Geometry: see drawing. Coordinates: mm, zero at the bounding-box minimum. Coordinates: 2 decimals unless noted, no trailing zeros. Order: outer loops, then holes, each group sorted by start corner. A loop starts at its lowest first (then second) coordinate and runs counter-clockwise, first axis right, second up.
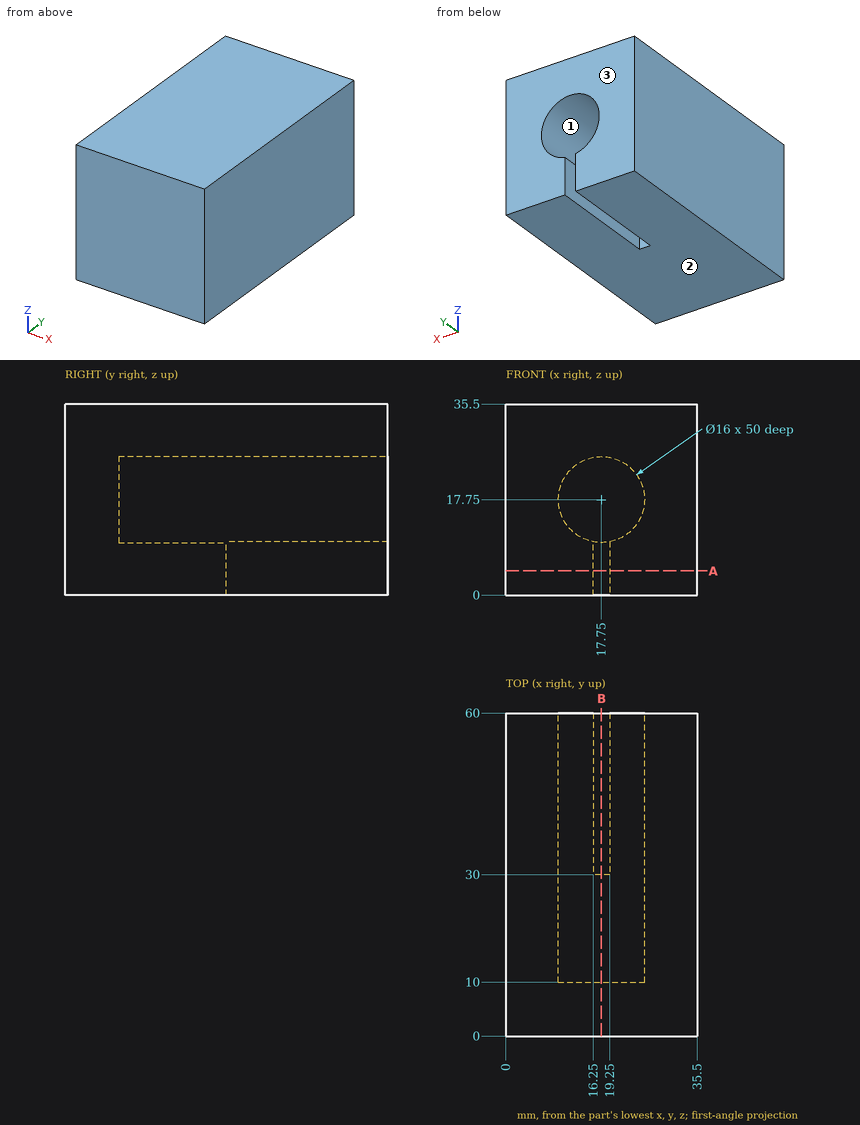
Q1. Section query B-B on x = 17.75. Output: boundary loops of the cut face in (y, z).
Solutions:
outline: (0, 0) - (30, 0) - (30, 9.75) - (10, 9.75) - (10, 25.75) - (60, 25.75) - (60, 35.5) - (0, 35.5) - close
Q2. Pull-direction query (Z, two-part tool) for the marked faces 1, 2 and 3; classes: pulls with the +Z half, pulls with the -Z half, needs draft (parallel to the pull), parting line crosses it, or undercut.
Solutions:
face 1: undercut
face 2: pulls with the -Z half
face 3: needs draft
Q3. Pin query (flat end, axial travel): P1, Ø5, axis at x = 19, z = 21, coming from the +Y side. Return the tip coordinate at first contact, or that it passes through.
Solutions:
P1: stops at y = 10
Q4. Material intervals for line 1 along X through (y, z) = (49.5, 17.75); line 2 along X through (y, z) = (31, 2); line 3 along Z through (x, y) = (17.75, 38), sorted ascending.
Solutions:
line 1: x = 0 to 9.75, 25.75 to 35.5
line 2: x = 0 to 16.25, 19.25 to 35.5
line 3: z = 25.75 to 35.5
Q5. Section query A-A on z = 4.5. Output: boundary loops of the cut face in (x, y), plus the area to 3 significant figures.
Solutions:
outline: (0, 0) - (35.5, 0) - (35.5, 60) - (19.25, 60) - (19.25, 30) - (16.25, 30) - (16.25, 60) - (0, 60) - close
area: 2,040 mm2
